```python
from build123d import *

# Parameters (mm, degrees)
SKETCH1_W            = 793.242
SKETCH1_H            = 571.5
BOSS_EXTRUDE1_DEPTH  = 25.4
FILLET1_R            = 17.78
SKETCH2_W            = 76.2
SKETCH2_H            = 25.4
BOSS_EXTRUDE2_DEPTH  = 58.42
FILLET2_R            = 12.7
SKETCH3_W            = 15.24
SKETCH3_H            = 38.1
CUT_EXTRUDE1_DEPTH   = 538.922423943
FILLET2_OF_MIRROR2_R = 12.7
SKETCH4_W            = 58.42
SKETCH4_H            = 25.4
BOSS_EXTRUDE3_DEPTH  = 50.8
FILLET3_R            = 22.86
FILLET4_R            = 22.86
SKETCH5_W            = 50.8
SKETCH5_H            = 15.24
CUT_EXTRUDE2_DEPTH   = 572.104596883
FILLET7_R            = 15.24
FILLET8_R            = 12.7


with BuildPart() as part:
    # Sketch1 → Boss-Extrude1 (new body)
    with BuildSketch(Plane(origin=(0, 0, 0), x_dir=(1, 0, 0), z_dir=(0, 1, 0))):
        Rectangle(SKETCH1_W, SKETCH1_H)
    boss_extrude1 = extrude(amount=BOSS_EXTRUDE1_DEPTH)

    # Fillet1
    fillet1_edges = [part.edges().sort_by_distance(p)[0] for p in [
        (0, 25.4, 285.75),
        (396.621, 12.7, 285.75),
        (-396.621, 12.7, 285.75),
        (-396.621, 12.7, -285.75),
        (396.621, 12.7, -285.75),
    ]]
    fillet(fillet1_edges, radius=FILLET1_R)

    # Sketch2 → Boss-Extrude2 (add)
    with BuildSketch(Plane.ZY.offset(396.621)):
        with Locations((-224.79, 12.7)):
            Rectangle(SKETCH2_W, SKETCH2_H)
    boss_extrude2 = extrude(amount=BOSS_EXTRUDE2_DEPTH)

    # Fillet2
    fillet2_edges = [part.edges().sort_by_distance(p)[0] for p in [
        (-455.041, 12.7, -262.89),
        (-455.041, 12.7, -186.69),
    ]]
    fillet(fillet2_edges, radius=FILLET2_R)

    # Sketch3 → Cut-Extrude1 (cut, through all)
    with BuildSketch(Plane(origin=(0, 25.4, 0), x_dir=(1, 0, 0), z_dir=(0, 1, 0))):
        with Locations((-435.991, 224.79)):
            Rectangle(SKETCH3_W, SKETCH3_H)
    cut_extrude1 = extrude(amount=-CUT_EXTRUDE1_DEPTH, mode=Mode.SUBTRACT)

    # Mirror2: Boss-Extrude1, Boss-Extrude2, Cut-Extrude1 across plane
    add(boss_extrude1.mirror(Plane(origin=(0, 0, 0), x_dir=(0, 0, 1), z_dir=(1, 0, 0))))
    add(boss_extrude2.mirror(Plane(origin=(0, 0, 0), x_dir=(0, 0, 1), z_dir=(1, 0, 0))))
    add(cut_extrude1.mirror(Plane(origin=(0, 0, 0), x_dir=(0, 0, 1), z_dir=(1, 0, 0))), mode=Mode.SUBTRACT)

    # Fillet2 of Mirror2
    fillet2_of_mirror2_edges = [part.edges().sort_by_distance(p)[0] for p in [
        (455.041, 12.7, -262.89),
        (455.041, 12.7, -186.69),
    ]]
    fillet(fillet2_of_mirror2_edges, radius=FILLET2_OF_MIRROR2_R)

    # Sketch4 → Boss-Extrude3 (add, symmetric)
    with BuildSketch(Plane(origin=(0, 0, 0), x_dir=(0, 0, -1), z_dir=(1, 0, 0))):
        with Locations((314.96, 12.7)):
            Rectangle(SKETCH4_W, SKETCH4_H)
    extrude(amount=BOSS_EXTRUDE3_DEPTH, both=True)

    # Fillet3
    fillet3_edges = [part.edges().sort_by_distance(p)[0] for p in [
        (396.621, 12.7, -285.75),
    ]]
    fillet(fillet3_edges, radius=FILLET3_R - 0.0001)  # a hair under: the kernel refuses the full size

    # Fillet4
    fillet4_edges = [part.edges().sort_by_distance(p)[0] for p in [
        (-396.621, 12.7, -285.75),
    ]]
    fillet(fillet4_edges, radius=FILLET4_R - 0.0001)  # a hair under: the kernel refuses the full size

    # Sketch5 → Cut-Extrude2 (cut, through all)
    with BuildSketch(Plane(origin=(0, 25.4, 0), x_dir=(1, 0, 0), z_dir=(0, 1, 0))):
        with Locations((0, 326.39)):
            Rectangle(SKETCH5_W, SKETCH5_H)
    extrude(amount=-CUT_EXTRUDE2_DEPTH, mode=Mode.SUBTRACT)

    # Fillet7
    fillet7_edges = [part.edges().sort_by_distance(p)[0] for p in [
        (-50.8, 12.7, -344.17),
        (50.8, 12.7, -344.17),
    ]]
    fillet(fillet7_edges, radius=FILLET7_R)

    # Fillet8
    fillet8_edges = [part.edges().sort_by_distance(p)[0] for p in [
        (0, 0, 285.75),
        (0, 25.4, 285.75),
        (-396.621, 12.7, 285.75),
        (396.621, 12.7, 285.75),
    ]]
    fillet(fillet8_edges, radius=FILLET8_R - 0.0001)  # a hair under: the kernel refuses the full size


solid = part.part
```
The model under review builds one solid part; all positions refer to its coordinate system, in mm. A direction names the side the tool comes from. Round coordinates to 2 decimals unless told otherwise and drop trailing zeros. Loops run counter-clockwise (first coordinate to the right, second up) from the corner with the lowest first, then second, coordinate; pieces in that order, holes last. Notation, with made-up numbers: (12.5, 87) - (64.5, 87) arc R17 ccw to (64.5, 106) - close; hole circle Ø6 at (45.25, 17.25). An arc over 180 degrees is marked (long way). Write each question's results on one line, items separated by ' | '. Start each with the question number.
Q1. Wall thickness on line 1 along X through (y, z) = (19.5, -217); line 2 along X through (y, z) = (11.75, -310.5); line 3 along Z through (x, y) = (247, 13.25): over which ranges is each line inside the solid? List them lowest first. Write a range as [from, to].
Q2. Take a section at C-C on z = -53. Give the boundary of the cut face in (x, y), plus the area to 3 significant figures.
Q3. Insertion check: P1, Ø7.5, axis at x = -186.5, y = 10.5, coming from the -Z side; P2, Ø4.5, axis at x = 433.5, y = 16.5, coming from the +Z side; P3, Ø12.5, axis at y = 12.5, z = -305.5, coming from the +X side. Each pin has a flat end and moves straight along its axis. Give the tip position at first contact, or say it passes through.
Q4. Take a section at A-A on z = -219.5. Give the boundary of the cut face in (x, y), plus the area to 3 significant figures.
Q5. Take a section at D-D on y = 21.5. Give the number of separate pieces and of enclosed holes in the cut face, plus the area to 3 significant figures.
Q6. Tool access review of faces 1 (the flat face through (-215, 13, -285.75)), 2 (the flat face through (-428.371, 13, -225)), 3 (the flat face through (50.8, 13, -307)): name each direction out of +Z, -Z, +X, -X, +Y, -Y from which nothing blocks a thin tool from reaching the whole face with its end or side.
Q7. Draft analysis for pull direction Z (two halves, no side actions). For faces 4 (the flat face through (6, 25.4, -40)), 5 (the flat face through (-443.611, 13, -225)), 6 (the flat face through (419, 13, -186.69)), state which applies: pulls with the +Z half, pulls with the -Z half, needs draft (parallel to the pull), parting line crosses it, or undercut.
Data:
1) line 1: x = [-455.04, -443.61], [-428.37, 428.37], [443.61, 455.04] | line 2: x = [-50.8, 50.8] | line 3: z = [-285.75, 285.74]
2) outline: (-396.62, 0) - (396.62, 0) - (396.62, 25.4) - (-396.62, 25.4) - close | area: 20,100 mm²
3) P1: stops at z = -285.75 | P2: stops at z = -186.69 | P3: stops at x = 50.8
4) outline: (-455.04, 0) - (-443.61, 0) - (-443.61, 25.4) - (-455.04, 25.4) - close; (-428.37, 0) - (428.37, 0) - (428.37, 25.4) - (-428.37, 25.4) - close; (443.61, 0) - (455.04, 0) - (455.04, 25.4) - (443.61, 25.4) - close | area: 22,300 mm²
5) separate pieces: 1 | enclosed holes: 3 | area: 463,000 mm²
6) face 1: -Z, -X, +Y, -Y | face 2: +Y, -Y | face 3: -Z, +X, +Y, -Y
7) face 4: needs draft | face 5: undercut | face 6: pulls with the +Z half
